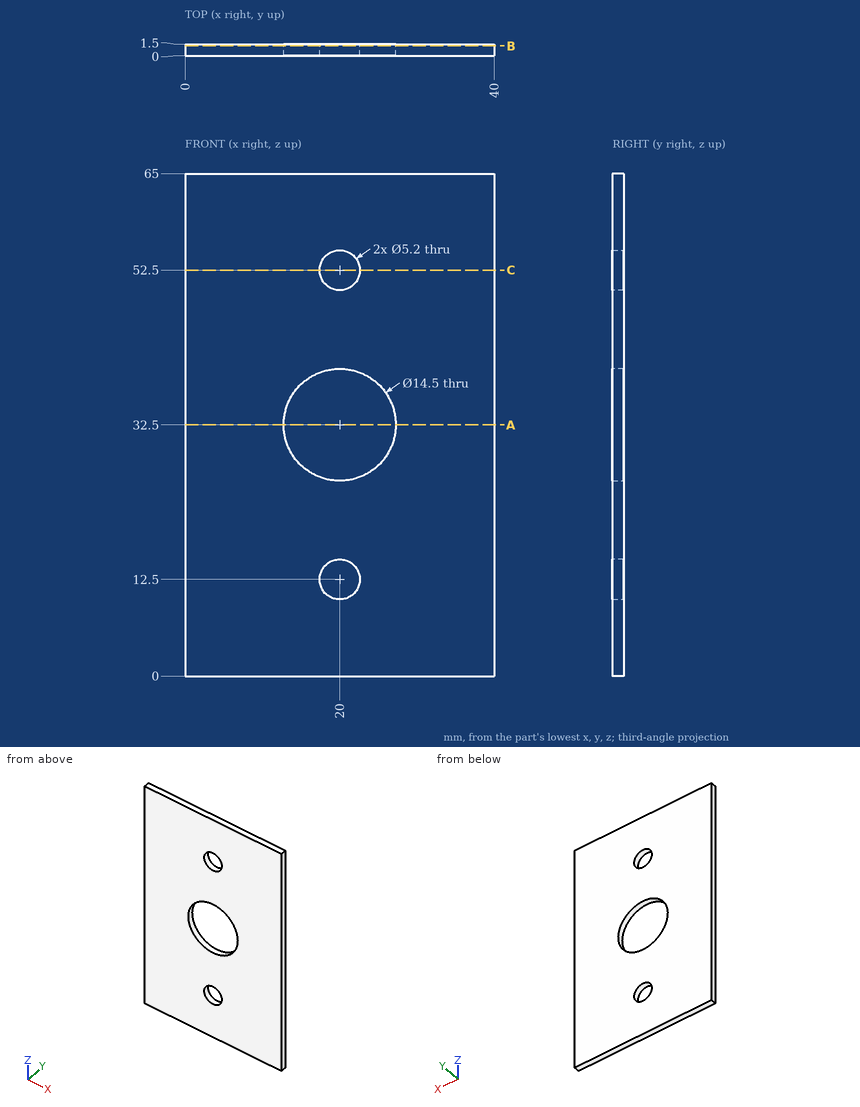
Design review of the part shown in the three views and the two pictorial views. Dimensions are in mm from the part's minimum x, y and z. Coordinates: 2 decimals unless noted, no trailing zeros. Loops run counter-clockwise (first coordinate to the right, second up) from the corner with the lowest first, then second, coordinate; pieces in that order, holes last.
(1) Wall thickness on L1, parallel to X at y = 0.55, z = 32.5; L2, parallel to X at y = 0.65, z = 52.5; L3, parallel to Z at x = 25, y = 0.2: over which ranges is each line inside the solid? List them lowest first.
Determined:
L1: x = 0 to 12.75, 27.25 to 40
L2: x = 0 to 17.4, 22.6 to 40
L3: z = 0 to 27.25, 37.75 to 65
(2) Consider section A-A, the plane z = 32.5. Give the boundary of the cut face in (x, y).
Determined:
outline: (0, 0) - (12.75, 0) - (12.75, 1.5) - (0, 1.5) - close; (27.25, 0) - (40, 0) - (40, 1.5) - (27.25, 1.5) - close
(3) Consider section C-C, the plane z = 52.5. Give the boundary of the cut face in (x, y).
Determined:
outline: (0, 0) - (17.4, 0) - (17.4, 1.5) - (0, 1.5) - close; (22.6, 0) - (40, 0) - (40, 1.5) - (22.6, 1.5) - close
(4) Consider section B-B, the plane y = 1.25. Give the boundary of the cut face in (x, z), plus the area to 3 significant figures.
Determined:
outline: (0, 0) - (40, 0) - (40, 65) - (0, 65) - close; hole circle Ø14.5 at (20, 32.5); hole circle Ø5.2 at (20, 12.5); hole circle Ø5.2 at (20, 52.5)
area: 2,390 mm2
(5) Insertion check: P1, Ø11.5, axis at x = 20, z = 32.5, coming from the -Y side. The pin has a flat end and moves straight along its axis. Give the tip position at first contact, or say it passes through.
Determined:
P1: passes through
